```python
from build123d import *

# Parameters (mm, degrees)
BOSS_EXTRUDE1_DEPTH     = 10
SKETCH3_R               = 1.5
CUT_EXTRUDE1_DEPTH      = 10
SKETCH5_R               = 1.525
SKETCH5_R_2             = 3.2
CUT_EXTRUDE2_DEPTH      = 10
FILLET1_R               = 1.2
CUT_EXTRUDE_THIN1_DEPTH = 5


with BuildPart() as part:
    # Sketch1 → Boss-Extrude1 (new body)
    with BuildSketch(Plane(origin=(0, 0, 0), x_dir=(1, 0, 0), z_dir=(0, 1, 0))):
        with BuildLine():
            Line((-90, -80), (90, -80))
            ThreePointArc((90, -80), (107.67766953, -72.67766953), (115, -55))
            Line((115, -55), (115, 55))
            ThreePointArc((115, 55), (107.67766953, 72.67766953), (90, 80))
            Line((90, 80), (-90, 80))
            ThreePointArc((-90, 80), (-107.67766953, 72.67766953), (-115, 55))
            Line((-115, 55), (-115, -55))
            ThreePointArc((-115, -55), (-107.67766953, -72.67766953), (-90, -80))
        make_face()
    extrude(amount=BOSS_EXTRUDE1_DEPTH)

    # Sketch3 → Cut-Extrude1 (cut)
    with BuildSketch(Plane(origin=(0, 10, 0), x_dir=(1, 0, 0), z_dir=(0, 1, 0))):
        with Locations(Location((-85, 50, 0), (0, 0, 270))):
            Circle(SKETCH3_R)
        with Locations(Location((85, 50, 0), (0, 0, 270))):
            Circle(SKETCH3_R)
        with Locations(Location((85, -50, 0), (0, 0, 270))):
            Circle(SKETCH3_R)
        with Locations(Location((-85, -50, 0), (0, 0, 270))):
            Circle(SKETCH3_R)
    extrude(amount=-CUT_EXTRUDE1_DEPTH, mode=Mode.SUBTRACT)

    # Sketch5 → Cut-Extrude2 (cut)
    with BuildSketch(Plane.XZ):
        with Locations(Location((23.52, -24.25, 0), (0, 0, 270))):
            Circle(SKETCH5_R)
        with Locations(Location((-23.52, -24.25, 0), (0, 0, 270))):
            Circle(SKETCH5_R)
        with Locations(Location((-39.598222878, 25, 0), (0, 0, 270))):
            Circle(SKETCH5_R_2)
        with Locations(Location((39.598222878, 25, 0), (0, 0, 270))):
            Circle(SKETCH5_R_2)
        Polygon((19.55, -20), (18.051220664, -28.5), (-18.051220664, -28.5), (-19.55, -20), align=None)
    extrude(amount=-CUT_EXTRUDE2_DEPTH, mode=Mode.SUBTRACT)

    # Fillet1
    fillet1_edges = [part.edges().sort_by_distance(p)[0] for p in [
        (-18.051220664, 5, -28.5),
        (-19.55, 5, -20),
        (19.55, 5, -20),
        (18.051220664, 5, -28.5),
    ]]
    fillet(fillet1_edges, radius=FILLET1_R)

    # Sketch7 → Cut-Extrude-Thin1 (cut)
    with BuildSketch(Plane.XZ):
        with BuildLine():
            Line((-85, 67.5), (85, 67.5))
            ThreePointArc((85, 67.5), (97.374368671, 62.374368671), (102.5, 50))
            Line((102.5, 50), (102.5, -50))
            ThreePointArc((102.5, -50), (97.374368671, -62.374368671), (85, -67.5))
            Line((85, -67.5), (-85, -67.5))
            ThreePointArc((-85, -67.5), (-97.374368671, -62.374368671), (-102.5, -50))
            Line((-102.5, -50), (-102.5, 50))
            ThreePointArc((-102.5, 50), (-97.374368671, 62.374368671), (-85, 67.5))
        make_face()
        with BuildLine():
            Line((-85, 62.5), (85, 62.5))
            ThreePointArc((85, 62.5), (93.838834765, 58.838834765), (97.5, 50))
            Line((97.5, 50), (97.5, -50))
            ThreePointArc((97.5, -50), (93.838834765, -58.838834765), (85, -62.5))
            Line((85, -62.5), (-85, -62.5))
            ThreePointArc((-85, -62.5), (-93.838834765, -58.838834765), (-97.5, -50))
            Line((-97.5, -50), (-97.5, 50))
            ThreePointArc((-97.5, 50), (-93.838834765, 58.838834765), (-85, 62.5))
        make_face(mode=Mode.SUBTRACT)
    extrude(amount=-CUT_EXTRUDE_THIN1_DEPTH, mode=Mode.SUBTRACT)


solid = part.part
```
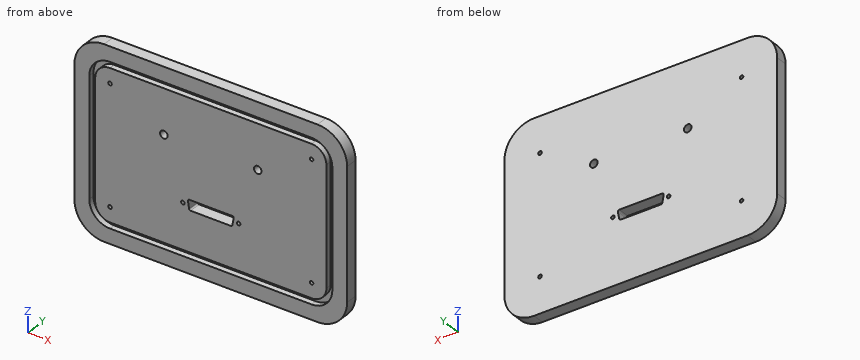
Geometry check sheet. Reference: the model listing, model coordinates, mm. Give positions to 0.01 mm unless a question says otherwise; leave off trailing zeros. Order: outer loops, then holes, each group sorted by start corner. A loop starts at its lowest first (then second) coordinate and runs counter-clockwise, first axis right, second up.
1. Section check A-A, the plane x = -6. Enter the section's corners in (y, z), and give its area (4 significant figures).
2. Thickness scan on L1, parallel to Z at x = 11, y = 3; L2, parallel to X at y = 2.25, z = 42; L3, parallel to X at y = 5.75, z = 50. Record the ranges inside material, lowest first.
3. Section check D-D, the plane x = -29. Enter the section's corners in (y, z), and give its area (3 significant figures).
4. Section check B-B, the plane z = 25. Enter the section's corners in (x, y), and give its area (3 significant figures).
5. Section check C-C, the plane y = 6.75. Give the number of separate pieces and of enclosed holes in the cut face, and give its area (3 significant figures).
Values follow:
1. outline: (0, -80) - (10, -80) - (10, -28.5) - (0, -28.5) - (0, -62.5) - (5, -62.5) - (5, -67.5) - (0, -67.5) - close; (0, -20) - (10, -20) - (10, 80) - (0, 80) - (0, 67.5) - (5, 67.5) - (5, 62.5) - (0, 62.5) - close
1. area: 1,465 mm2
2. L1: z = -80 to -67.5, -62.5 to -28.5, -20 to 62.5, 67.5 to 80
2. L2: x = -115 to -102.5, -97.5 to 97.5, 102.5 to 115
2. L3: x = -115 to -86.5, -83.5 to 83.5, 86.5 to 115
3. outline: (0, -80) - (10, -80) - (10, 80) - (0, 80) - (0, 67.5) - (5, 67.5) - (5, 62.5) - (0, 62.5) - (0, -62.5) - (5, -62.5) - (5, -67.5) - (0, -67.5) - close
3. area: 1,550 mm2
4. outline: (-115, 0) - (-102.5, 0) - (-102.5, 5) - (-97.5, 5) - (-97.5, 0) - (-42.8, 0) - (-42.8, 10) - (-115, 10) - close; (-36.4, 0) - (36.4, 0) - (36.4, 10) - (-36.4, 10) - close; (42.8, 0) - (97.5, 0) - (97.5, 5) - (102.5, 5) - (102.5, 0) - (115, 0) - (115, 10) - (42.8, 10) - close
4. area: 2,120 mm2
5. separate pieces: 1
5. enclosed holes: 9
5. area: 35,800 mm2
